Design review of the part shown in the three views and the two pictorial views. Dimensions are in mm from the part's minimum x, y and z. A direction names the side the tool comes from. Round coordinates to 2 decimals unless told otherwise and drop trailing zeros. Order: outer loops, then holes, each group sorted by start corner. A loop starts at its lowest first (then second) coordinate and runs counter-clockwise, first axis right, second up.
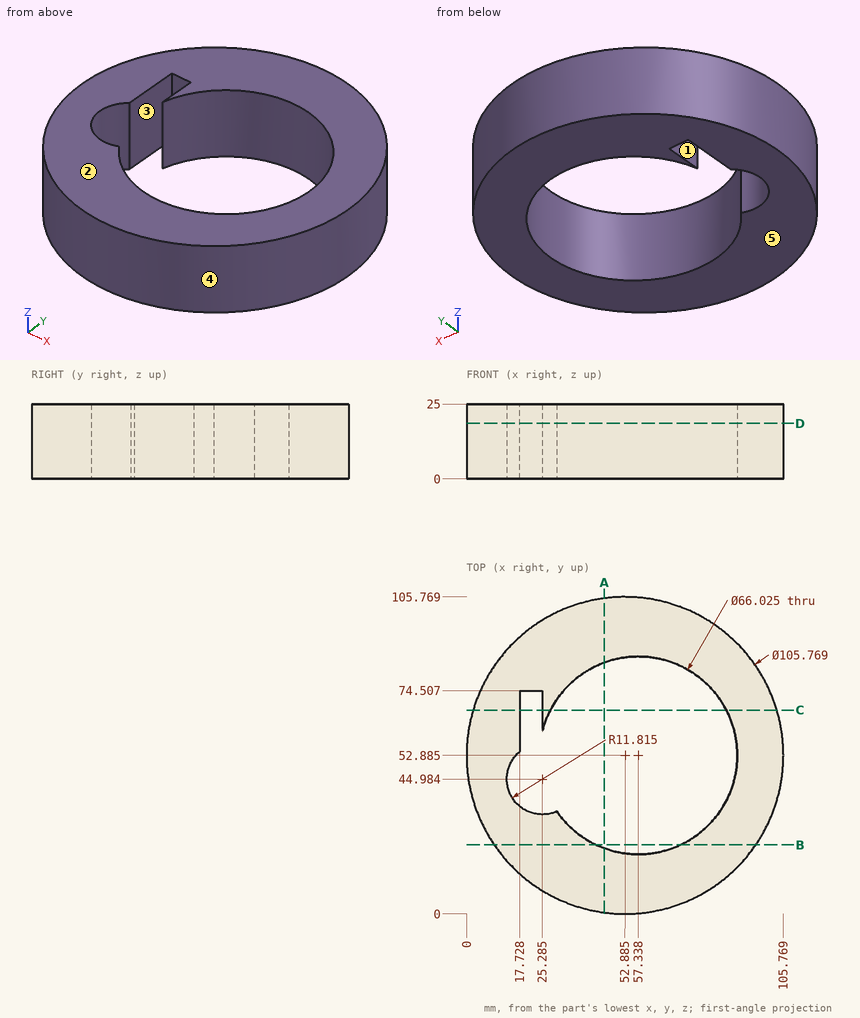
1) To check wall thickness, follow line 1 along X through (y, z) = (62.5, 17.25) (1 decimal); line 2 along Y through (x, z) = (50, 3); line 3 along Y through (x, z) = (47, 14.25) (1 decimal). State the ranges of each line that lie inside material, in increasing order.
Results:
line 1: x = 0.9 to 17.7, 25.3 to 25.8, 88.9 to 104.9
line 2: y = 0.08 to 20.7, 85.07 to 105.69
line 3: y = 0.3 to 21.5, 84.2 to 105.4
2) The part is to be moulded in two halves that separate along X. For the marked faces 3, 4 and 5, say which applies: released by +X, released by -X, zero draft, split by the parting line, or undercut.
Results:
face 3: undercut
face 4: split by the parting line
face 5: zero draft
3) Take a section at D-D on z = 18.5. Give the boundary of the cut face in (x, y) (1 decimal), plus the area to 3 significant figures.
Results:
outline: circle Ø105.8 at (52.9, 52.9); hole (17.7, 54.1) arc R11.8 ccw to (30.1, 34.2) arc R33 ccw (long way) to (25.3, 60.8) - (25.3, 74.5) - (17.7, 74.5) - close
area: 4,990 mm2
4) Take a section at A-A on x = 46. Give the boundary of the cut face in (y, z), plus the area to 3 significant figures.
Results:
outline: (0.45, 0) - (21.88, 0) - (21.88, 25) - (0.45, 25) - close; (83.89, 0) - (105.32, 0) - (105.32, 25) - (83.89, 25) - close
area: 1,070 mm2
5) Take a section at C-C on y = 68. Give the boundary of the cut face in (x, z) (1 decimal).
Results:
outline: (2.2, 0) - (17.7, 0) - (17.7, 25) - (2.2, 25) - close; (25.3, 0) - (28, 0) - (28, 25) - (25.3, 25) - close; (86.7, 0) - (103.6, 0) - (103.6, 25) - (86.7, 25) - close
6) For the marked faces 1 and 2, list the 3-axis set-ups (+Z, -Z, +X, -X, +Y, -Y) from which the entire face can be reached by the end or side of a thin tool; tool diameter is ignored.
Results:
face 1: +Z, -Z
face 2: +Z, +X, -X, +Y, -Y
7) Clearance check with flat-ended pins moving along their axes: P1, Ø6, axis at x = 29, z = 16.5, coming from the -Y side; P2, Ø1, axis at y = 78, z = 3.5, coming from the -X side; P3, Ø6, axis at y = 67.5, z = 17, coming from the +X side. State where each tip first meets the part, or that it passes through.
Results:
P1: stops at y = 4.3
P2: stops at x = 6.08
P3: stops at x = 104.48
8) Take a section at B-B on y = 23. Give the boundary of the cut face in (x, z) (1 decimal).
Results:
outline: (9.3, 0) - (43.3, 0) - (43.3, 25) - (9.3, 25) - close; (71.4, 0) - (96.5, 0) - (96.5, 25) - (71.4, 25) - close
